```python
from build123d import *

# Parameters (mm, degrees)
PAD_DEPTH       = 14
POCKET_DEPTH    = 12
SKETCH020_W     = 77.5
SKETCH020_H     = 38.5
POCKET010_DEPTH = 2
SKETCH021_W     = 3.5
SKETCH021_H     = 5
PAD004_DEPTH    = 4
SKETCH022_W     = 3.5
SKETCH022_H     = 5
PAD005_DEPTH    = 4
SKETCH023_W     = 3.5
SKETCH023_H     = 5
PAD006_DEPTH    = 4
SKETCH024_R     = 2
PAD007_DEPTH    = 5
PAD008_DEPTH    = 5
PAD009_DEPTH    = 10
SKETCH027_W     = 13
SKETCH027_H     = 13
POCKET011_DEPTH = 2
SKETCH028_R     = 0.7
HOLE_DEPTH      = 3.579398
HOLE_TIPS_R     = 0.7
SKETCH029_R     = 0.7
HOLE001_DEPTH   = 3.579398
HOLE001_TIPS_R  = 0.7
SKETCH030_R     = 18.5
POCKET012_DEPTH = 1
FILLET_R        = 3
FILLET001_R     = 2
FILLET002_R     = 1
FILLET003_R     = 2
FILLET004_R     = 1
FILLET005_R     = 1


with BuildPart() as part:
    # Sketch → Pad (new body)
    with BuildSketch(Plane.XY):
        with BuildLine():
            Line((0, 0), (0, 42.5))
            Line((0, 42.5), (-85, 42.5))
            Line((-85, 42.5), (-117.747865, 15.410813))
            ThreePointArc((-117.747865, 15.410813), (-113.515965, -18.096324), (-85, 0))
            Line((0, 0), (-85, 0))
        make_face()
    extrude(amount=PAD_DEPTH)

    # Sketch019 (on Face6 of Pad) → Pocket (cut)
    with BuildSketch(Plane(origin=(0, 0, 0), x_dir=(1, 0, 0), z_dir=(0, 0, -1))):
        with BuildLine():
            Line((-116.570177, -13.7888), (-84.28, -40.5))
            Line((-84.28, -40.5), (-2, -40.5))
            Line((-2, -40.5), (-2, -2))
            Line((-2, -2), (-87, -2))
            Line((-87, -2), (-87, 0))
            ThreePointArc((-87, 0), (-112.607129, 16.31354), (-116.570177, -13.7888))
        make_face()
    extrude(amount=-POCKET_DEPTH, mode=Mode.SUBTRACT)

    # Sketch020 (on Face5 of Pocket) → Pocket010 (cut)
    with BuildSketch(Plane.XY.offset(14)):
        with Locations((-40.75, 21.25)):
            Rectangle(SKETCH020_W, SKETCH020_H)
    extrude(amount=-POCKET010_DEPTH, mode=Mode.SUBTRACT)

    # Sketch021 (on Face12 of Pocket010) → Pad004 (join)
    with BuildSketch(Plane.XZ.offset(-40.5)):
        with Locations((-21.25, 9.5)):
            Rectangle(SKETCH021_W, SKETCH021_H)
        with Locations((-60.25, 9.5)):
            Rectangle(SKETCH021_W, SKETCH021_H)
    extrude(amount=PAD004_DEPTH)

    # Sketch022 (on Face10 of Pad004) → Pad005 (join)
    with BuildSketch(Plane(origin=(0, 2, 0), x_dir=(-1, 0, 0), z_dir=(0, 1, 0))):
        with Locations((21.25, 9.5)):
            Rectangle(SKETCH022_W, SKETCH022_H)
        with Locations((60.25, 9.5)):
            Rectangle(SKETCH022_W, SKETCH022_H)
        with Locations((40.75, 4.5)):
            Rectangle(SKETCH022_W, SKETCH022_H)
    extrude(amount=PAD005_DEPTH)

    # Sketch023 (on Face11 of Pad005) → Pad006 (join)
    with BuildSketch(Plane(origin=(-2, 0, 0), x_dir=(0, -1, 0), z_dir=(-1, 0, 0))):
        with Locations((-21.25, 4.5)):
            Rectangle(SKETCH023_W, SKETCH023_H)
    extrude(amount=PAD006_DEPTH)

    # Sketch024 (on Face18 of Pad006) → Pad007 (join)
    with BuildSketch(Plane(origin=(0, 0, 12), x_dir=(1, 0, 0), z_dir=(0, 0, -1))):
        with Locations((-93, 0)):
            Circle(SKETCH024_R)
        with Locations((-117, 0)):
            Circle(SKETCH024_R)
        with Locations((-105, -12)):
            Circle(SKETCH024_R)
        with BuildLine():
            ThreePointArc((-88.636932, 7.5), (-105, 18), (-121.363068, 7.5))
            Line((-121.363068, 7.5), (-88.636932, 7.5))
        make_face()
    extrude(amount=PAD007_DEPTH)

    # Sketch025 (on Face20 of Pad007) → Pad008 (join)
    with BuildSketch(Plane(origin=(0, 0, 7), x_dir=(1, 0, 0), z_dir=(0, 0, -1))):
        with BuildLine():
            ThreePointArc((-92.5501, 13), (-105, 18), (-117.4499, 13))
            Line((-117.4499, 13), (-92.5501, 13))
        make_face()
    extrude(amount=PAD008_DEPTH)

    # Sketch026 (on Face18 of Pad008) → Pad009 (join)
    with BuildSketch(Plane(origin=(0, 0, 12), x_dir=(1, 0, 0), z_dir=(0, 0, -1))):
        Polygon((-100, -27.5), (-90, -27.5), (-90, -35.77), align=None)
    extrude(amount=PAD009_DEPTH)

    # Sketch027 (on Face18 of Pad009) → Pocket011 (cut)
    with BuildSketch(Plane(origin=(0, 0, 12), x_dir=(1, 0, 0), z_dir=(0, 0, -1))):
        with Locations((-105, 0)):
            Rectangle(SKETCH027_W, SKETCH027_H)
    extrude(amount=-POCKET011_DEPTH, mode=Mode.SUBTRACT)

    # Sketch028 (on Face42 of Pocket011) → Hole (cut)
    with BuildSketch(Plane(origin=(0, 0, 7), x_dir=(1, 0, 0), z_dir=(0, 0, -1))):
        with Locations((-60.25, -4)):
            Circle(SKETCH028_R)
        with Locations((-21.25, -4)):
            Circle(SKETCH028_R)
        with Locations((-21.25, -38.5)):
            Circle(SKETCH028_R)
        with Locations((-60.25, -38.5)):
            Circle(SKETCH028_R)
        with Locations((-105, -12)):
            Circle(SKETCH028_R)
        with Locations((-93, 0)):
            Circle(SKETCH028_R)
        with Locations((-117, 0)):
            Circle(SKETCH028_R)
        with Locations((-105, 10)):
            Circle(SKETCH028_R)
    extrude(amount=-HOLE_DEPTH, mode=Mode.SUBTRACT)

    # Hole tips → Hole tip 1 section 0
    with BuildSketch(Plane(origin=(0, 0, 10.579398), x_dir=(1, 0, 0), z_dir=(0, 0, -1)), mode=Mode.PRIVATE) as hole_tip_1_s0:
        with Locations((-60.25, -4)):
            Circle(HOLE_TIPS_R)
    loft([hole_tip_1_s0.sketch, Vertex(-60.25, 4, 11)], mode=Mode.SUBTRACT)

    # Hole tips → Hole tip 2 section 0
    with BuildSketch(Plane(origin=(0, 0, 10.579398), x_dir=(1, 0, 0), z_dir=(0, 0, -1)), mode=Mode.PRIVATE) as hole_tip_2_s0:
        with Locations((-21.25, -4)):
            Circle(HOLE_TIPS_R)
    loft([hole_tip_2_s0.sketch, Vertex(-21.25, 4, 11)], mode=Mode.SUBTRACT)

    # Hole tips → Hole tip 3 section 0
    with BuildSketch(Plane(origin=(0, 0, 10.579398), x_dir=(1, 0, 0), z_dir=(0, 0, -1)), mode=Mode.PRIVATE) as hole_tip_3_s0:
        with Locations((-21.25, -38.5)):
            Circle(HOLE_TIPS_R)
    loft([hole_tip_3_s0.sketch, Vertex(-21.25, 38.5, 11)], mode=Mode.SUBTRACT)

    # Hole tips → Hole tip 4 section 0
    with BuildSketch(Plane(origin=(0, 0, 10.579398), x_dir=(1, 0, 0), z_dir=(0, 0, -1)), mode=Mode.PRIVATE) as hole_tip_4_s0:
        with Locations((-60.25, -38.5)):
            Circle(HOLE_TIPS_R)
    loft([hole_tip_4_s0.sketch, Vertex(-60.25, 38.5, 11)], mode=Mode.SUBTRACT)

    # Hole tips → Hole tip 5 section 0
    with BuildSketch(Plane(origin=(0, 0, 10.579398), x_dir=(1, 0, 0), z_dir=(0, 0, -1)), mode=Mode.PRIVATE) as hole_tip_5_s0:
        with Locations((-105, -12)):
            Circle(HOLE_TIPS_R)
    loft([hole_tip_5_s0.sketch, Vertex(-105, 12, 11)], mode=Mode.SUBTRACT)

    # Hole tips → Hole tip 6 section 0
    with BuildSketch(Plane(origin=(0, 0, 10.579398), x_dir=(1, 0, 0), z_dir=(0, 0, -1)), mode=Mode.PRIVATE) as hole_tip_6_s0:
        with Locations((-93, 0)):
            Circle(HOLE_TIPS_R)
    loft([hole_tip_6_s0.sketch, Vertex(-93, 0, 11)], mode=Mode.SUBTRACT)

    # Hole tips → Hole tip 7 section 0
    with BuildSketch(Plane(origin=(0, 0, 10.579398), x_dir=(1, 0, 0), z_dir=(0, 0, -1)), mode=Mode.PRIVATE) as hole_tip_7_s0:
        with Locations((-117, 0)):
            Circle(HOLE_TIPS_R)
    loft([hole_tip_7_s0.sketch, Vertex(-117, 0, 11)], mode=Mode.SUBTRACT)

    # Hole tips → Hole tip 8 section 0
    with BuildSketch(Plane(origin=(0, 0, 10.579398), x_dir=(1, 0, 0), z_dir=(0, 0, -1)), mode=Mode.PRIVATE) as hole_tip_8_s0:
        with Locations((-105, 10)):
            Circle(HOLE_TIPS_R)
    loft([hole_tip_8_s0.sketch, Vertex(-105, -10, 11)], mode=Mode.SUBTRACT)

    # Sketch029 (on Face48 of Hole) → Hole001 (cut)
    with BuildSketch(Plane(origin=(0, 0, 2), x_dir=(1, 0, 0), z_dir=(0, 0, -1))):
        with Locations((-105, 15)):
            Circle(SKETCH029_R)
        with Locations((-93, -30)):
            Circle(SKETCH029_R)
        with Locations((-40.75, -4)):
            Circle(SKETCH029_R)
        with Locations((-4, -21.25)):
            Circle(SKETCH029_R)
    extrude(amount=-HOLE001_DEPTH, mode=Mode.SUBTRACT)

    # Hole001 tips → Hole001 tip 1 section 0
    with BuildSketch(Plane(origin=(0, 0, 5.579398), x_dir=(1, 0, 0), z_dir=(0, 0, -1)), mode=Mode.PRIVATE) as hole001_tip_1_s0:
        with Locations((-105, 15)):
            Circle(HOLE001_TIPS_R)
    loft([hole001_tip_1_s0.sketch, Vertex(-105, -15, 6)], mode=Mode.SUBTRACT)

    # Hole001 tips → Hole001 tip 2 section 0
    with BuildSketch(Plane(origin=(0, 0, 5.579398), x_dir=(1, 0, 0), z_dir=(0, 0, -1)), mode=Mode.PRIVATE) as hole001_tip_2_s0:
        with Locations((-93, -30)):
            Circle(HOLE001_TIPS_R)
    loft([hole001_tip_2_s0.sketch, Vertex(-93, 30, 6)], mode=Mode.SUBTRACT)

    # Hole001 tips → Hole001 tip 3 section 0
    with BuildSketch(Plane(origin=(0, 0, 5.579398), x_dir=(1, 0, 0), z_dir=(0, 0, -1)), mode=Mode.PRIVATE) as hole001_tip_3_s0:
        with Locations((-40.75, -4)):
            Circle(HOLE001_TIPS_R)
    loft([hole001_tip_3_s0.sketch, Vertex(-40.75, 4, 6)], mode=Mode.SUBTRACT)

    # Hole001 tips → Hole001 tip 4 section 0
    with BuildSketch(Plane(origin=(0, 0, 5.579398), x_dir=(1, 0, 0), z_dir=(0, 0, -1)), mode=Mode.PRIVATE) as hole001_tip_4_s0:
        with Locations((-4, -21.25)):
            Circle(HOLE001_TIPS_R)
    loft([hole001_tip_4_s0.sketch, Vertex(-4, 21.25, 6)], mode=Mode.SUBTRACT)

    # Sketch030 (on Face5 of Hole001) → Pocket012 (cut)
    with BuildSketch(Plane.XY.offset(14)):
        with Locations((-105, 0)):
            Circle(SKETCH030_R)
    extrude(amount=-POCKET012_DEPTH, mode=Mode.SUBTRACT)

    # Fillet
    fillet_edges = [part.edges().sort_by_distance(p)[0] for p in [
        (0, 0, 7),
        (0, 42.5, 7),
        (-85, 42.5, 7),
        (-85, 0, 7),
    ]]
    fillet(fillet_edges, radius=FILLET_R)

    # Fillet001
    fillet001_edges = [part.edges().sort_by_distance(p)[0] for p in [
        (-2, 40.5, 13),
        (-2, 2, 13),
        (-79.5, 40.5, 13),
        (-79.5, 2, 13),
    ]]
    fillet(fillet001_edges, radius=FILLET001_R)

    # Fillet002
    fillet002_edges = [part.edges().sort_by_distance(p)[0] for p in [
        (-62, 2, 9.5),
        (-62, 6, 9.5),
        (-58.5, 6, 9.5),
        (-58.5, 2, 9.5),
        (-42.5, 2, 4.5),
        (-42.5, 6, 4.5),
        (-39, 6, 4.5),
        (-39, 2, 4.5),
        (-23, 6, 9.5),
        (-19.5, 6, 9.5),
        (-19.5, 2, 9.5),
        (-23, 2, 9.5),
        (-19.5, 40.5, 9.5),
        (-19.5, 36.5, 9.5),
        (-23, 36.5, 9.5),
        (-62, 36.5, 9.5),
        (-58.5, 36.5, 9.5),
        (-58.5, 40.5, 9.5),
        (-62, 40.5, 9.5),
        (-23, 40.5, 9.5),
        (-6, 19.5, 4.5),
        (-6, 23, 4.5),
        (-2, 19.5, 4.5),
        (-2, 23, 4.5),
    ]]
    fillet(fillet002_edges, radius=FILLET002_R)

    # Fillet003
    fillet003_edges = [part.edges().sort_by_distance(p)[0] for p in [
        (-88.636932, -7.5, 9.5),
        (-121.363068, -7.5, 9.5),
        (-92.5501, -13, 4.5),
        (-117.4499, -13, 4.5),
        (-84.28, 40.5, 6),
        (-99.995217, 27.5, 7),
        (-90, 35.76828, 7),
        (-90, 27.5, 7),
    ]]
    fillet(fillet003_edges, radius=FILLET003_R)

    # Fillet004
    fillet004_edges = [part.edges().sort_by_distance(p)[0] for p in [
        (-111.5, 6.5, 12.5),
        (-98.5, -6.5, 12.5),
        (-111.5, -6.5, 12.5),
        (-98.5, 6.5, 12.5),
    ]]
    fillet(fillet004_edges, radius=FILLET004_R)

    # Fillet005
    fillet005_edges = [part.edges().sort_by_distance(p)[0] for p in [
        (-119, 0, 12),
        (-107, 12, 12),
        (-95, 0, 12),
    ]]
    fillet(fillet005_edges, radius=FILLET005_R)


solid = part.part
```
Design review of the part built by this model. Coordinates are the model's own, in mm. A direction names the side the tool comes from. Coordinates: 2 decimals unless noted, no trailing zeros. Loops run counter-clockwise (first coordinate to the right, second up) from the corner with the lowest first, then second, coordinate; pieces in that order, holes last. Notation, with made-up numbers: (-36.5, 2.25) - (22.5, 2.25) arc R28 ccw to (22.5, 36.25) - close; hole circle Ø3 at (50, 65.25). An arc over 180 degrees is marked (long way). Use CSV: the item, a comma, the result in double quotes. Start each with the question number.
1) Wall thickness on L1, parallel to Y at x = -41, z = 8.75; L2, parallel to X at y = 38.5, z = 9.15; L3, parallel to Y at x = -93.5, z = 3: over which ranges is each line inside the solid? List them lowest first. Write a range as from..to.
2) Tool access review of faces 5 (the flat face through (-60, 39, 12)), 6 (the flat face through (-104, 12, 7)), 7 (the flat face through (-81, 21, 14)): name each direction out of +Z, -Z, +X, -X, +Y, -Y from which nothing blocks a thin tool from reaching the whole face with its end or side.
3) Consider section A-A on x = -53.5. Write out the cut boundary in (y, z).
4) The part is to be moulded in two halves that separate along X. For faces 1 (the cylindrical face through (-91.092, -0.601, 9.028)), 2 (the cylindrical face through (-84.152, -0.725, 7.098)), 3 (the flat face through (-21, 39, 12)), 4 (the flat face through (-43, 42.5, 7)), say which applies: +X half, -X half, draft (parallel to the pull), parting line (faces both ways), or undercut.
5) For pin 1 Ø8 at (y, z) = (-1.5, 10) entering from +X; pin 2 Ø3 at (x, y) = (-20, 4.5) entering from -Z; pin 3 Ø3 at (x, y) = (-20, 38) entering from +Z, all flat-tipped, find the tip position at first contact; note any pin that passes through.
Geometry says:
1,L1,"0..2, 40.5..42.5"
1,L2,"-89.84..-86.7, -62..-60.95, -59.55..-58.5, -23..-21.95, -20.55..-19.5, -2..0"
1,L3,"-16.36..-13, 27.5..29.51, 30.49..35.47"
2,face 5,"+Z"
2,face 6,"-Z"
2,face 7,"+Z, +X, -X, +Y, -Y"
3,outline,"(0, 0) - (2, 0) - (2, 14) - (0, 14) - close; (40.5, 0) - (42.5, 0) - (42.5, 14) - (40.5, 14) - close"
4,face 1,"undercut"
4,face 2,"+X half"
4,face 3,"undercut"
4,face 4,"draft"
5,pin 1,"x = -0.04"
5,pin 2,"z = 7"
5,pin 3,"z = 12"
